Check sheet for the drawn part. Datum: minimum x, y, z corner. Units: mm. Give positions to 0.01 mm unless a question says otherwise; leave off trailing zeros. Loops run counter-clockwise (first coordinate to the right, second up) from the corner with the lowest first, then second, coordinate; pieces in that order, holes last. Notation, with made-up numbers: (-16.5, 41.5) - (-0.5, 41.5) arc R36 cw to (-0.5, 77.5) - close; hole circle Ø8 at (38, 67.25). An arc over 180 degrees is marked (long way). One line per item, written item: value. Start each with the question number.
1. Sectioned sample at B-B (z = 1.3). Count the separate pieces of the cut face and the enclosed holes in it, plus the area to 3 significant figures.
2. Sectioned sample at A-A (y = 11.43). Record the cut outline in (x, z).
3. Gauge pin test, flat end, axial feed: pin 1 (3 mm diameter, centred on x = 9.017, y = 88.9, fed in from -Z). Record the tip position at first contact, or that the pin passes through.
4. Sectioned sample at C-C (x = 5.5). Record the cut outline in (y, z).
5. Scan lines: L1, parallel to Y at x = 12.5, z = 1.45; L2, parallel to Y at x = 5.5, z = 0.8; L3, parallel to X at y = 56.5, z = 1.1 (3 decimals). Record each from-to range of solid material in increasing order. Write a range as [from, to].
6. Sectioned sample at D-D (y = 88.9). Record the cut outline in (x, z).
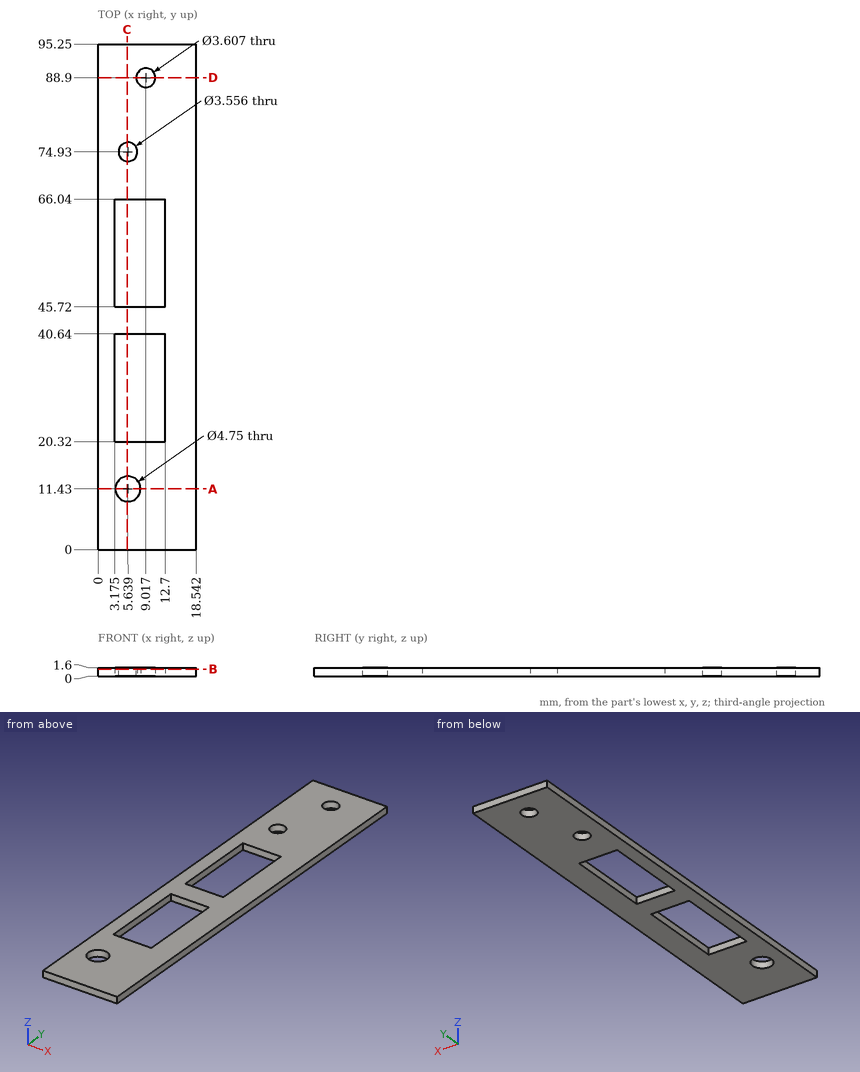
Results are:
1. separate pieces: 1
1. enclosed holes: 5
1. area: 1,340 mm^2
2. outline: (0, 0) - (3.26, 0) - (3.26, 1.6) - (0, 1.6) - close; (8.01, 0) - (18.54, 0) - (18.54, 1.6) - (8.01, 1.6) - close
3. pin 1: passes through
4. outline: (0, 0) - (9.06, 0) - (9.06, 1.6) - (0, 1.6) - close; (13.8, 0) - (20.32, 0) - (20.32, 1.6) - (13.8, 1.6) - close; (40.64, 0) - (45.72, 0) - (45.72, 1.6) - (40.64, 1.6) - close; (66.04, 0) - (73.16, 0) - (73.16, 1.6) - (66.04, 1.6) - close; (76.7, 0) - (95.25, 0) - (95.25, 1.6) - (76.7, 1.6) - close
5. L1: y = [0, 20.32], [40.64, 45.72], [66.04, 95.25]
5. L2: y = [0, 9.06], [13.8, 20.32], [40.64, 45.72], [66.04, 73.16], [76.7, 95.25]
5. L3: x = [0, 3.175], [12.7, 18.542]
6. outline: (0, 0) - (7.21, 0) - (7.21, 1.6) - (0, 1.6) - close; (10.82, 0) - (18.54, 0) - (18.54, 1.6) - (10.82, 1.6) - close
